Verification items for the finished model (mm, model axes). Face numbers are marked on the shaded views. A direction names the side the tool comes from. Coordinates: 2 decimals unless noted, no trailing zeros. Loops run counter-clockwise (first coordinate to the right, second up) from the corner with the lowest first, then second, coordinate; pieces in that order, holes last. Notation, with made-up numbers: (-13, -24.75) -> (15, -24.75) arc R21 cw to (15, -4.75) -> close; hole circle Ø3 at (-22.75, -13.75). An arc over 180 degrees is marked (long way). Answer as a JSON object with one key per item and string values. Group by question number.
Q1. Gauge pin test, flat ends, axial feed: pin 1 Ø4.5 at (x, y) = (2, 8.5) entering from +Z; pin 2 Ø3.5 at (y, z) = (-34, 6) entering from -X; pin 3 Ø10 at (x, z) = (-12.5, 2.5) entering from -Y. Record the tip position at first contact, or that the pin passes through.
Q2. Release check for a two-part mould opening along Y. For the marked faces 1, 2, 3 and 4 record: released by +Y, released by -Y, zero draft, split by the parting line, or undercut.
Q3. Set-up check for the marked faces 5, 6, 7 and 8: record each of +Z, -Z, +X, -X, +Y, -Y from which the full face is reachable in a straight line by a thin tool's end or side.
Q4. Scan lines: L1, parallel to Y at x = 10, z = 6 (3 decimals); L2, parallel to Y at x = 14, z = 6; L3, parallel to X at y = 8, z = 17. Record each from-to range of solid material in increasing order.
Q5. Cross-section at C-C on y = -34. Record the boundary of the cut face in (x, z) (3 decimals).
Q6. Cross-section at B-B on z = 6. Record the boundary of the cut face in (x, y) (3 decimals), and give its area (3 significant figures).
Q7. Cross-section at D-D on x = -10. Record the boundary of the cut face in (y, z), and give its area (3 significant figures).
Q8. Cross-section at A-A on y = -44. Record the boundary of the cut face in (x, z), and give its area (3 significant figures).
```python
from build123d import *

# Parameters (mm, degrees)
SKETCH_1_W          = 30
SKETCH_1_H          = 39.8
EXTRUDE_1_DEPTH     = 4
SKETCH_2_W          = 30
SKETCH_2_H          = 14
EXTRUDE_2_DEPTH     = 9
SKETCH_3_W          = 30
SKETCH_3_H          = 6
EXTRUDE_3_DEPTH     = 9
SKETCH_4_W          = 10
SKETCH_4_H          = 39.8
EXTRUDE_4_DEPTH     = 60
SKETCH_5_W          = 20
SKETCH_5_H          = 10
CUT_EXTRUDE_1_DEPTH = 70.971494196
SKETCH_6_W          = 3.9
SKETCH_6_H          = 6
CUT_EXTRUDE_2_DEPTH = 70.971494196
SKETCH_8_W          = 12
SKETCH_8_H          = 4
EXTRUDE_5_DEPTH     = 30
SKETCH_9_W          = 12
SKETCH_9_H          = 7.651073012
SKETCH_9_H_2        = 46.348926988
EXTRUDE_6_DEPTH     = 10
SKETCH_13_R         = 1.6
SKETCH_13_R_2       = 1.615
CUT_EXTRUDE_3_DEPTH = 71.835090174
SKETCH_14_R         = 3
CUT_EXTRUDE_4_DEPTH = 2
CUT_EXTRUDE_5_REACH = 75.546
SKETCH_16_R         = 2.05
SKETCH_18_R         = 2.05
CUT_EXTRUDE_7_DEPTH = 71.835090174
STOPPER_DEPTH       = 4.6


with BuildPart() as part:
    # 草图1 → 凸台-拉伸1 (new body)
    with BuildSketch(Plane(origin=(0, 0, 0), x_dir=(1, 0, 0), z_dir=(0, 1, 0))):
        Rectangle(SKETCH_1_W, SKETCH_1_H)
    extrude(amount=EXTRUDE_1_DEPTH)

    # 草图2 → 凸台-拉伸2 (add)
    with BuildSketch(Plane(origin=(0, 4, 0), x_dir=(1, 0, 0), z_dir=(0, 1, 0))):
        with Locations((0, 12.9)):
            Rectangle(SKETCH_2_W, SKETCH_2_H)
    extrude(amount=EXTRUDE_2_DEPTH)

    # 草图3 → 凸台-拉伸3 (add)
    with BuildSketch(Plane(origin=(0, 4, 0), x_dir=(1, 0, 0), z_dir=(0, 1, 0))):
        with Locations((0, -16.9)):
            Rectangle(SKETCH_3_W, SKETCH_3_H)
    extrude(amount=EXTRUDE_3_DEPTH)

    # 草图4 → 凸台-拉伸4 (add)
    with BuildSketch(Plane(origin=(0, 0, 0), x_dir=(-1, 0, 0), z_dir=(0, -1, 0))):
        with Locations((-10, 0)):
            Rectangle(SKETCH_4_W, SKETCH_4_H)
    extrude(amount=EXTRUDE_4_DEPTH)

    # 草图5 → 切除-拉伸1 (cut, through all)
    with BuildSketch(Plane(origin=(15, 0, 0), x_dir=(0, 0, -1), z_dir=(1, 0, 0))):
        with Locations((-6, -11)):
            Rectangle(SKETCH_5_W, SKETCH_5_H)
    extrude(amount=-CUT_EXTRUDE_1_DEPTH, mode=Mode.SUBTRACT)

    # 草图6 → 切除-拉伸2 (cut, through all)
    with BuildSketch(Plane(origin=(15, 0, 0), x_dir=(0, 0, -1), z_dir=(1, 0, 0))):
        with Locations((-17.95, -10.651073012)):
            Rectangle(SKETCH_6_W, SKETCH_6_H)
    extrude(amount=-CUT_EXTRUDE_2_DEPTH, mode=Mode.SUBTRACT)

    # 草图8 → 凸台-拉伸5 (add)
    with BuildSketch(Plane.ZY.offset(15)):
        with Locations((25.9, 2)):
            Rectangle(SKETCH_8_W, SKETCH_8_H)
    extrude(amount=-EXTRUDE_5_DEPTH)

    # 草图9 → 凸台-拉伸6 (add)
    with BuildSketch(Plane.ZY.offset(-5)):
        with Locations((25.9, -3.825536506)):
            Rectangle(SKETCH_9_W, SKETCH_9_H)
        with Locations((25.9, -36.825536506)):
            Rectangle(SKETCH_9_W, SKETCH_9_H_2)
    extrude(amount=-EXTRUDE_6_DEPTH)

    # 草图13 → 切除-拉伸3 (cut, through all)
    with BuildSketch(Plane.ZY.offset(-5)):
        with Locations((-4, -44)):
            Circle(SKETCH_13_R)
        with Locations((6, -34)):
            Circle(SKETCH_13_R_2)
        with Locations((16, -44)):
            Circle(SKETCH_13_R)
        with Locations((6, -54)):
            Circle(SKETCH_13_R)
    extrude(amount=-CUT_EXTRUDE_3_DEPTH, mode=Mode.SUBTRACT)

    # 草图14 → 切除-拉伸4 (cut)
    with BuildSketch(Plane(origin=(15, 0, 0), x_dir=(0, 0, -1), z_dir=(1, 0, 0))):
        with Locations((-6, -34)):
            Circle(SKETCH_14_R)
        with Locations((-16, -44)):
            Circle(SKETCH_14_R)
        with Locations((-6, -54)):
            Circle(SKETCH_14_R)
        with Locations((4, -44)):
            Circle(SKETCH_14_R)
    extrude(amount=-CUT_EXTRUDE_4_DEPTH, mode=Mode.SUBTRACT)

    # 草图16 → 切除-拉伸5 (cut, up to next)
    with BuildSketch(Plane.XY.offset(19.9), mode=Mode.PRIVATE) as cut_extrude_5_sk1:
        with Locations((-10, 8.5)):
            Circle(SKETCH_16_R)
    cut_extrude_5_tool1 = extrude(cut_extrude_5_sk1.sketch, amount=-CUT_EXTRUDE_5_REACH, mode=Mode.PRIVATE) & part.part
    # 草图16 → 切除-拉伸5 (cut, up to next)
    with BuildSketch(Plane.XY.offset(19.9), mode=Mode.PRIVATE) as cut_extrude_5_sk2:
        with Locations((0, 8.5)):
            Circle(SKETCH_16_R)
    cut_extrude_5_tool2 = extrude(cut_extrude_5_sk2.sketch, amount=-CUT_EXTRUDE_5_REACH, mode=Mode.PRIVATE) & part.part
    # 草图16 → 切除-拉伸5 (cut, up to next)
    with BuildSketch(Plane.XY.offset(19.9), mode=Mode.PRIVATE) as cut_extrude_5_sk3:
        with Locations((10, 8.5)):
            Circle(SKETCH_16_R)
    cut_extrude_5_tool3 = extrude(cut_extrude_5_sk3.sketch, amount=-CUT_EXTRUDE_5_REACH, mode=Mode.PRIVATE) & part.part
    add(cut_extrude_5_tool1.solids().sort_by_distance((-10, 8.5, 19.9))[0], mode=Mode.SUBTRACT)
    add(cut_extrude_5_tool2.solids().sort_by_distance((0, 8.5, 19.9))[0], mode=Mode.SUBTRACT)
    add(cut_extrude_5_tool3.solids().sort_by_distance((10, 8.5, 19.9))[0], mode=Mode.SUBTRACT)

    # 草图18 → 切除-拉伸7 (cut, through all)
    with BuildSketch(Plane.ZY.offset(-5)):
        with Locations((23.95, -4.151073012)):
            Circle(SKETCH_18_R)
        with Locations((23.95, -17.151073012)):
            Circle(SKETCH_18_R)
    extrude(amount=-CUT_EXTRUDE_7_DEPTH, mode=Mode.SUBTRACT)

    # 草图21 → Stopper (add)
    with BuildSketch(Plane.ZY.offset(15)):
        Polygon((31.9, 0), (31.9, 4), (19.9, 4), (19.9, 13), (13.9, 13), (13.9, 4), (-5.9, 4), (-5.9, 13), (-19.9, 13), (-19.9, 0), align=None)
    extrude(amount=STOPPER_DEPTH)


solid = part.part
```
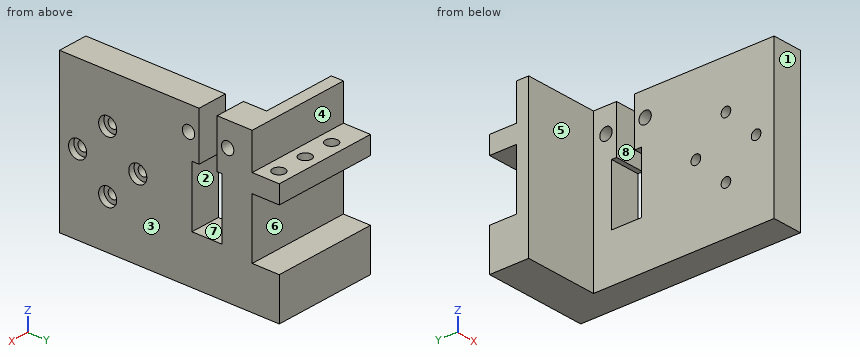
Computed values:
{
 "1": {"pin 1": "stops at z = 19.9", "pin 2": "stops at x = 5", "pin 3": "stops at y = 0"},
 "2": {"face 1": "released by -Y", "face 2": "undercut", "face 3": "zero draft", "face 4": "released by +Y"},
 "3": {"face 5": "+Z, -Z, -X, -Y", "face 6": "+X, -X, +Y", "face 7": "+X, -X", "face 8": "+Z, +X, -X"},
 "4": {"L1": "y = -60 to -55.6, -52.4 to -35.615, -32.385 to -16, -6 to 4", "L2": "y = -60 to -57, -51 to -37, -31 to -16, -6 to 4", "L3": "x = -19.6 to -11.99, -8.01 to -1.99, 1.99 to 8.01, 11.99 to 15"},
 "5": {"outline": "(5, -19.9) -> (15, -19.9) -> (15, 3) -> (13, 3) -> (13, 4.385) -> (5, 4.385) -> close; (5, 7.615) -> (13, 7.615) -> (13, 9) -> (15, 9) -> (15, 31.9) -> (5, 31.9) -> close"},
 "6": {"outline": "(-19.6, 0) -> (5, 0) -> (5, -6) -> (15, -6) -> (15, 4) -> (-19.6, 4) -> close; (5, -60) -> (15, -60) -> (15, -57) -> (13, -57) -> (13, -55.6) -> (5, -55.6) -> close; (5, -52.4) -> (13, -52.4) -> (13, -51) -> (15, -51) -> (15, -37) -> (13, -37) -> (13, -35.615) -> (5, -35.615) -> close; (5, -32.385) -> (13, -32.385) -> (13, -31) -> (15, -31) -> (15, -16) -> (5, -16) -> close", "area": "563 mm²"},
 "7": {"outline": "(0, -19.9) -> (13, -19.9) -> (13, -5.9) -> (4, -5.9) -> (4, 13.9) -> (6.45, 13.9) -> (6.45, 19.9) -> (4, 19.9) -> (4, 31.9) -> (0, 31.9) -> close; (10.55, 13.9) -> (13, 13.9) -> (13, 19.9) -> (10.55, 19.9) -> close", "area": "363 mm²"},
 "8": {"outline": "(5, -19.9) -> (15, -19.9) -> (15, -7) -> (13, -7) -> (13, -5.6) -> (5, -5.6) -> close; (5, -2.4) -> (13, -2.4) -> (13, -1) -> (15, -1) -> (15, 13) -> (13, 13) -> (13, 14.4) -> (5, 14.4) -> close; (5, 17.6) -> (13, 17.6) -> (13, 19) -> (15, 19) -> (15, 31.9) -> (5, 31.9) -> close", "area": "443 mm²"}
}
